Here's how the part is built. I have some questions about the finished solid (model axes, mm). A direction names the side the tool comes from. Round coordinates to 2 decimals unless told otherwise and drop trailing zeros. Loops run counter-clockwise (first coordinate to the right, second up) from the corner with the lowest first, then second, coordinate; pieces in that order, holes last. Notation, with made-up numbers: (39, -10.5) - (48, -10.5) arc R21 ccw to (48, -5.5) - close; hole circle Ø10 at (-17, -35.5). An arc over 180 degrees is marked (long way). Answer as a JSON object with one key per item and string values. Group by question number.
1) I want a section at B-B, the plane z = 0.5. Please give me the cut outline in (x, y).
2) Will these pins go through, and if not, where does the flat tip stop? P1, Ø8, axis at y = -3.5, z = 11.5, coming from the -X side; P2, Ø12, axis at x = 3, y = 3.5, coming from the +Z side; P3, Ø0.7, axis at x = 8.5, y = -3, coming from the -Z side; P4, Ø1.9, axis at y = -3, z = 1.5, coming from the -X side.
3) If I drill on line 1 along X through (y, z) = (-0.75, 20.5); line 2 along Y through (x, z) = (-0.25, 12.5); line 3 along Z through (x, y) = (7.5, 14.5), over which ranges is the centre line in solid material (lowest first)? Write a range as [from, to].
4) I want a section at C-C, the plane x = -0.5. Please give me the cut outline in (y, z).
5) Which directions (+Z, -Z, +X, -X, +Y, -Y) give clear straight access to the entire face, cutting with the end or side of a thin tool? Please do faces 4 (the face through (-3.257, 14.411, 26.496)), 5 (the face through (-8.4, -3, 0)), 6 (the face through (-9, -3, 0)), 7 (the face through (3.243, 14.389, 26.496)).
6) I want a section at A-A, the plane y = -3.5. Please give me the cut outline in (x, z), then the cut area to 3 significant figures.
7) If we mould it in two halves opening along X, with no side actions, what happens to faces 1 (the face through (9, -3, 0)), 2 (the face through (8.4, -3, 0)), 3 (the face through (0, 8, 26.25))? For each: pulls with the +X half, pulls with the -X half, needs draft (parallel to the pull), parting line crosses it, or undercut.
8) I want a section at D-D, the plane x = -6.75. Please give me the cut outline in (y, z), then the cut area to 4 significant figures.
from build123d import *

# Parameters (mm, degrees)
SKETCH1_W           = 21
SKETCH1_H           = 52.5
BOSS_EXTRUDE1_DEPTH = 16.6
BOSS_EXTRUDE2_DEPTH = 0.5
SKETCH3_W           = 0.6
SKETCH3_H           = 49.5
BOSS_EXTRUDE3_DEPTH = 6.4


with BuildPart() as part:
    # Sketch1 → Boss-Extrude1 (new body)
    with BuildSketch(Plane(origin=(0, 0, 0), x_dir=(1, 0, 0), z_dir=(0, 1, 0))):
        Rectangle(SKETCH1_W, SKETCH1_H)
    extrude(amount=BOSS_EXTRUDE1_DEPTH)

    # Sketch2 → Boss-Extrude2 (add)
    with BuildSketch(Plane.XY.offset(26.25)):
        Polygon((-3.75, 16.6), (-3.75, 15.2), (-2.75, 13.6), (2.75, 13.6), (3.75, 15.2), (3.75, 16.6), align=None)
    extrude(amount=BOSS_EXTRUDE2_DEPTH)

    # Sketch3 → Boss-Extrude3 (add)
    with BuildSketch(Plane.XZ):
        with Locations((-8.7, 0)):
            Rectangle(SKETCH3_W, SKETCH3_H)
        with Locations((8.7, 0)):
            Rectangle(SKETCH3_W, SKETCH3_H)
    extrude(amount=BOSS_EXTRUDE3_DEPTH)


solid = part.part
Outcome:
{
 "1": {"outline": "(-10.5, 0) - (-9, 0) - (-9, -6.4) - (-8.4, -6.4) - (-8.4, 0) - (8.4, 0) - (8.4, -6.4) - (9, -6.4) - (9, 0) - (10.5, 0) - (10.5, 16.6) - (-10.5, 16.6) - close"},
 "2": {"P1": "x = -10.5", "P2": "z = 26.25", "P3": "z = -24.75", "P4": "x = -9"},
 "3": {"line 1": "[-9, -8.4], [8.4, 9]", "line 2": "[0, 16.6]", "line 3": "[-26.25, 26.25]"},
 "4": {"outline": "(0, -26.25) - (16.6, -26.25) - (16.6, 26.75) - (13.6, 26.75) - (13.6, 26.25) - (0, 26.25) - close"},
 "5": {"face 4": "+Z, -X, -Y", "face 5": "+Z, -Z, -Y", "face 6": "+Z, -Z, -X, -Y", "face 7": "+Z, +X, -Y"},
 "6": {"outline": "(-9, -24.75) - (-8.4, -24.75) - (-8.4, 24.75) - (-9, 24.75) - close; (8.4, -24.75) - (9, -24.75) - (9, 24.75) - (8.4, 24.75) - close", "area": "59.4 mm^2"},
 "7": {"face 1": "pulls with the +X half", "face 2": "undercut", "face 3": "needs draft"},
 "8": {"outline": "(0, -26.25) - (16.6, -26.25) - (16.6, 26.25) - (0, 26.25) - close", "area": "871.5 mm^2"}
}
